Part model, mm, in its own coordinate system. A direction names the side the tool comes from. Round coordinates to 2 decimals unless told otherwise and drop trailing zeros. Write each loop counter-clockwise with the first axis right and the second up, starting at its lowest first coordinate (ties: lowest second). Pieces come first, ordered by that corner, then holes. Notation, with made-up numbers: (49.5, 63) -> (98.5, 63) arc R25 cw to (98.5, 102) -> close; hole circle Ø5 at (35.25, -0.5). An arc over 180 degrees is marked (long way). Return JSON: item names as keys, results as strings. Group by question number.
(1) Drill centre lines: L1, parallel to Z at x = -233.5, y = -32 (3 decimals); L2, parallel to Y at x = -131.5, z = 9.25; L3, parallel to X at y = 69.5, z = 2. Where is each one in solid material? Low to high. Write a range as from..to.
(2) Saw through at B-B (y = 13). List the corners of the cut face in (x, z) (3 decimals).
(3) Mould opens along Y. For faces 3 (the flat face through (-92, -10, 24.895)), 4 (the flat face through (-142.831, 45.926, 13.525)), 5 (the flat face through (-119.2, -35, 0)), 6 (the cylindrical face through (-284.267, -72.822, 13.525)) say: +Y half, -Y half, draft (parallel to the pull), parting line (faces both ways), or undercut.
(4) Drop flat-ended pins along their axis: pin 1 Ø1.5 at (y, z) = (-30, 9.5) entering from -X; pin 2 Ø6 at (y, z) = (-31, 3) entering from -X; pin 3 Ø1.5 at (y, z) = (33, 18) entering from +X; pin 4 Ø5 at (x, y) = (-131.39, 2.59) entering from +Z. Give the stop position or say it passes through.
(5) Tool access for faces 1 (the flat face through (-92, -10, 27.435)), 2 (the flat face through (-101.224, -105.168, 12.273)): list every direction of +Z, -Z, +X, -X, +Y, -Y with a clear straight run to the whole face (end or side of a thin tool).
(6) Saw through at A-A (z = 19). State how many separate pieces and enclosed holes the cut face has, plus the area to 3 significant figures.
(7) Saw through at C-C (x = 0). List the corners of the cut face in (y, z) (3 decimals).
from build123d import *

# Parameters (mm, degrees)
SKETCH1_R           = 3.175
BOSS_EXTRUDE1_DEPTH = 27.435
SHELL1_T            = -2.54


with BuildPart() as part:
    # Sketch1 → Boss-Extrude1 (new body)
    with BuildSketch(Plane.XY):
        with BuildLine():
            Line((-246.406013588, 3.788089061), (-36.31395184, 89.260287536))
            ThreePointArc((-36.31395184, 89.260287536), (93.454251213, 23.503296779), (10.232750038, -95.819584929))
            Line((10.232750038, -95.819584929), (-215.29793902, -119.904422791))
            ThreePointArc((-215.29793902, -119.904422791), (-284.593997313, -71.574027866), (-246.406013588, 3.788089061))
        make_face()
        with Locations(Location((-131.38650471, 2.593989183, 0), (0, 0, 180))):
            Circle(SKETCH1_R, mode=Mode.SUBTRACT)
        with Locations(Location((-116.729233004, -32.575302177, 0), (0, 0, 180))):
            Circle(SKETCH1_R, mode=Mode.SUBTRACT)
        with Locations(Location((-122.41902156, -97.213498796, 0), (0, 0, 180))):
            Circle(SKETCH1_R, mode=Mode.SUBTRACT)
    extrude(amount=BOSS_EXTRUDE1_DEPTH)

    # Shell1
    shell1_openings = [part.faces().sort_by_distance(p)[0] for p in [
        (-83.986643927, -21.103730923, 0),
    ]]
    offset(amount=SHELL1_T, openings=shell1_openings, kind=Kind.INTERSECTION)


solid = part.part
Computed values:
{
 "1": {"L1": "24.895..27.435", "L2": "-110.96..-108.4, -3.12..-0.58, 5.77..8.31, 47.79..50.54", "L3": "-84.89..-78.14, 63.03..66.75"},
 "2": {"outline": "(-223.763, 0) -> (-217.023, 0) -> (-217.023, 24.895) -> (92.919, 24.895) -> (92.919, 0) -> (95.484, 0) -> (95.484, 27.435) -> (-223.763, 27.435) -> close"},
 "3": {"face 3": "undercut", "face 4": "+Y half", "face 5": "draft", "face 6": "parting line"},
 "4": {"pin 1": "x = -281.44", "pin 2": "x = -282.71", "pin 3": "x = 90.81", "pin 4": "through"},
 "5": {"face 1": "+Z, +X, -X, +Y, -Y", "face 2": "-Z"},
 "6": {"separate pieces": "4", "enclosed holes": "4", "area": "2,650 mm2"},
 "7": {"outline": "(-96.912, 0) -> (-94.358, 0) -> (-94.358, 24.895) -> (93.824, 24.895) -> (93.824, 0) -> (96.364, 0) -> (96.364, 27.435) -> (-96.912, 27.435) -> close"}
}
